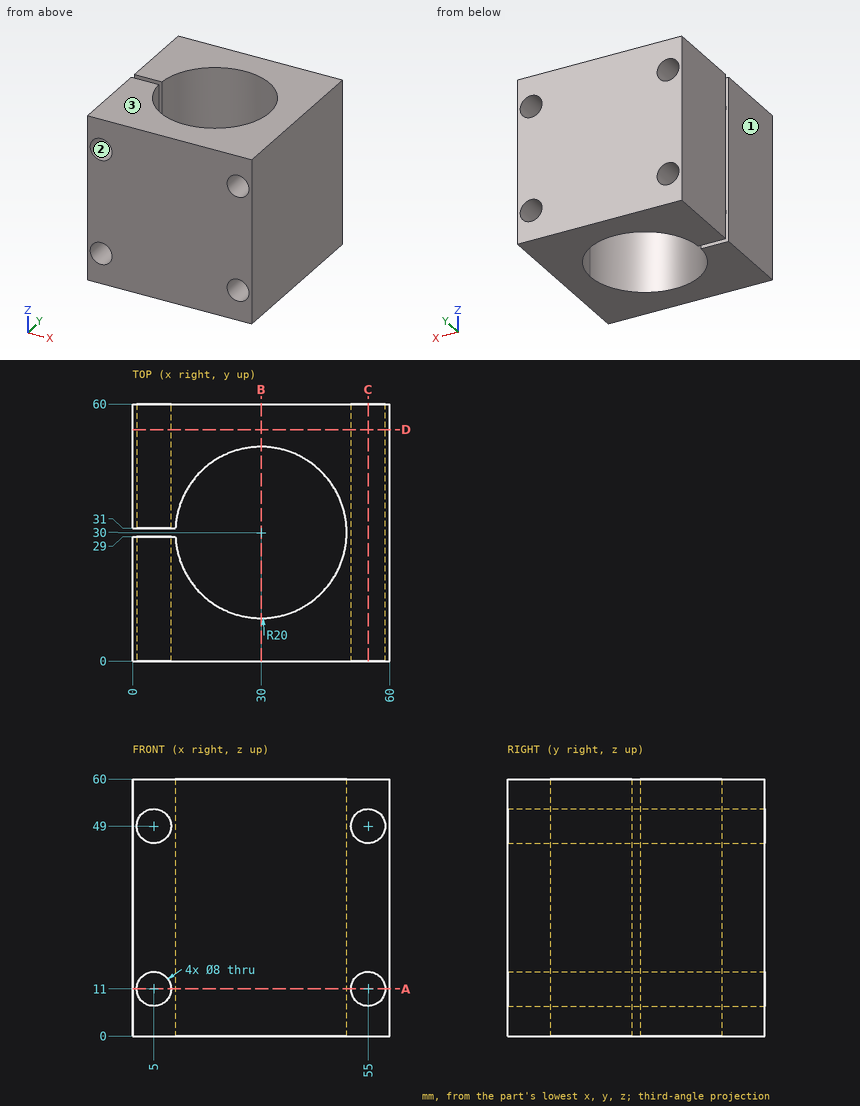
Drawing for the job (mm, zero at the part's lowest x, y, z). Round coordinates to 2 decimals unless told otherwise and drop trailing zeros. Loops run counter-clockwise (first coordinate to the right, second up) from the corner with the lowest first, then second, coordinate; pieces in that order, holes last. Notation, with made-up numbers: M 45,23 L 68,23 A5 cw 68,31 Z; hole C -29.75,81 d4. An arc over 180 degrees is marked long. Use a Markdown table: item, result. Add a question column.
(1) Cut at C-C (x = 55). Give the cut face in (y, z).
(2) Drill centre lines: line 1 (Z direction, x = 5, y = 21.75); line 2 (Z direction, x = 54, y = 38); line 3 (X direction, y = 12, z = 12). Where is each one in solid material? Low to high.
(3) Pull direction X, two halves, no side cores. Call the marked faces 1, 2 and 3: +X half, -X half, draft (parallel to the pull), parting line (faces both ways), or undercut.
(4) Cut at B-B (x = 30). Give the cut face in (y, z).
(5) Cut at D-D (y = 54). Give the cut face in (x, z), and give its area (3 significant figures).
(6) Cut at A-A (z = 11). Give the cut face in (x, y), and give its area (3 significant figures).
(7) Flat gauge pin, fed straight in: pin 1 (10 mm diameter, centred on x = 31, y = 42, fed in from +Z). Where does the tip first touch, or does it go through?
Geometry says:
| question | item | result |
|---|---|---|
| 1 | outline | M 0,0 L 60,0 L 60,7 L 0,7 Z; M 0,15 L 60,15 L 60,45 L 0,45 Z; M 0,53 L 60,53 L 60,60 L 0,60 Z |
| 2 | line 1 | z = 0 to 7, 15 to 45, 53 to 60 |
| 2 | line 2 | z = 0 to 7.13, 14.87 to 45.13, 52.87 to 60 |
| 2 | line 3 | x = 0 to 1.13, 8.87 to 21.28, 38.72 to 51.13, 58.87 to 60 |
| 3 | face 1 | -X half |
| 3 | face 2 | undercut |
| 3 | face 3 | draft |
| 4 | outline | M 0,0 L 10,0 L 10,60 L 0,60 Z; M 50,0 L 60,0 L 60,60 L 50,60 Z |
| 5 | outline | M 0,0 L 60,0 L 60,60 L 0,60 Z; hole C 5,11 d8; hole C 5,49 d8; hole C 55,11 d8; hole C 55,49 d8 |
| 5 | area | 3,400 mm² |
| 6 | outline | M 0,0 L 1,0 L 1,29 L 0,29 Z; M 0,31 L 1,31 L 1,60 L 0,60 Z; M 9,0 L 51,0 L 51,60 L 9,60 L 9,31 L 10.03,31 A20 cw long 10.03,29 L 9,29 Z; M 59,0 L 60,0 L 60,60 L 59,60 Z |
| 6 | area | 1,380 mm² |
| 7 | pin 1 | passes through |
